The model under review builds one solid part; all positions refer to its coordinate system, in mm. Give positions to 0.01 mm unless a question says otherwise; leave off trailing zeros. Order: outer loops, then holes, each group sorted by start corner. A loop starts at its lowest first (then second) coordinate and runs counter-clockwise, first axis right, second up. Notation, with made-up numbers: (-34, 25.5) - (-8, 25.5) arc R37 cw to (-8, 62.5) - close; hole circle Ø11 at (67, 2.25). An arc over 180 degrees is marked (long way). Write item = value, one per line. Start each with the question number.
1. We need section B-B, the plane z = -0.6. State how many separate pieces and enclosed holes the cut face has, and give its area (3 significant figures).
2. For P1, Ø1.9, axis at x = -138.08, y = 6.57, coming from the -Z side; P2, Ø1.5, axis at x = 94.5, z = 0.5, coming from the -Y side; P3, Ø5, axis at x = 138.08, y = 6.57, coming from the -Z side; P4, Ø1.5, axis at x = 75, z = 0, coming from the +Y side, all flat-tipped, find the tip position at first contact; note any pin that passes through.
3. Wall thickness on probe 1 along Y at (x, z) = (49, 0.8); probe 2 along X at (y, z) = (-22.5, 0.15); probe 3 along Y at (x, z) = (-219, 1.2): over which ranges is each line inside the solid? List them lowest first.
4. We need section A-A, the plane y = -38.5. Give the boundary of the cut face in (x, z), and give its area (3 significant figures).
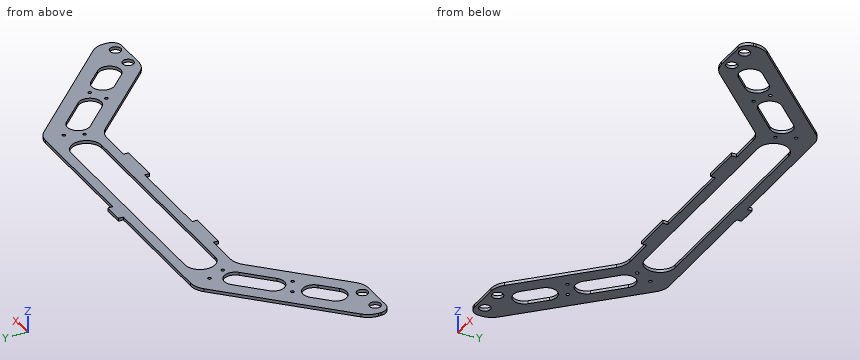
from build123d import *

# Parameters (mm, degrees)
SKETCH_1_R          = 5.5
EXTRUDE_1_DEPTH     = 1.5
CUT_EXTRUDE_6_DEPTH = 283.134941999
SKETCH_2_5_R        = 1.6
CUT_EXTRUDE_7_DEPTH = 283.134941999


with BuildPart() as part:
    # Sketch 1 → Extrude 1 (new, symmetric)
    with BuildSketch(Plane.XY):
        with BuildLine():
            Line((-125, 25), (-10, 25))
            Line((-10, 25), (-10, 30))
            Line((-10, 30), (10, 30))
            Line((10, 30), (10, 25))
            Line((10, 25), (125, 25))
            Line((125, 25), (137.426406871, 25))
            ThreePointArc((137.426406871, 25), (145.080075518, 23.47759065), (151.568542495, 19.142135624))
            Line((151.568542495, 19.142135624), (202.781745931, -32.071067812))
            Line((202.781745931, -32.071067812), (253.994949366, -83.284271247))
            ThreePointArc((253.994949366, -83.284271247), (258.330404393, -89.772738224), (259.852813742, -97.426406871))
            Line((259.852813742, -97.426406871), (259.852813742, -99.852813742))
            ThreePointArc((259.852813742, -99.852813742), (256.923881554, -106.923881554), (249.852813742, -109.852813742))
            Line((249.852813742, -109.852813742), (218.13708499, -109.852813742))
            ThreePointArc((218.13708499, -109.852813742), (210.483416343, -108.330404393), (203.994949366, -103.994949366))
            Line((203.994949366, -103.994949366), (130.857864376, -30.857864376))
            ThreePointArc((130.857864376, -30.857864376), (124.3693974, -26.52240935), (116.715728753, -25))
            Line((116.715728753, -25), (85, -25))
            Line((85, -25), (85, -30))
            Line((85, -30), (45, -30))
            Line((45, -30), (45, -25))
            Line((45, -25), (-45, -25))
            Line((-45, -25), (-45, -30))
            Line((-45, -30), (-85, -30))
            Line((-85, -30), (-85, -25))
            Line((-85, -25), (-116.715728753, -25))
            ThreePointArc((-116.715728753, -25), (-124.3693974, -26.52240935), (-130.857864376, -30.857864376))
            Line((-130.857864376, -30.857864376), (-203.994949366, -103.994949366))
            ThreePointArc((-203.994949366, -103.994949366), (-210.483416343, -108.330404393), (-218.13708499, -109.852813742))
            Line((-218.13708499, -109.852813742), (-249.852813742, -109.852813742))
            ThreePointArc((-249.852813742, -109.852813742), (-256.923881554, -106.923881554), (-259.852813742, -99.852813742))
            Line((-259.852813742, -99.852813742), (-259.852813742, -97.426406871))
            ThreePointArc((-259.852813742, -97.426406871), (-258.330404393, -89.772738224), (-253.994949366, -83.284271247))
            Line((-253.994949366, -83.284271247), (-202.781745931, -32.071067812))
            Line((-202.781745931, -32.071067812), (-151.568542495, 19.142135624))
            ThreePointArc((-151.568542495, 19.142135624), (-145.080075518, 23.47759065), (-137.426406871, 25))
            Line((-137.426406871, 25), (-125, 25))
        make_face()
        with Locations((-245.994949366, -101.352813742)):
            Circle(SKETCH_1_R, mode=Mode.SUBTRACT)
        with Locations((-221.994949366, -101.352813742)):
            Circle(SKETCH_1_R, mode=Mode.SUBTRACT)
        with Locations((221.994949366, -101.352813742)):
            Circle(SKETCH_1_R, mode=Mode.SUBTRACT)
        with Locations((245.994949366, -101.352813742)):
            Circle(SKETCH_1_R, mode=Mode.SUBTRACT)
    extrude(amount=EXTRUDE_1_DEPTH, both=True)

    # Sketch 2 → Cut-Extrude 6 (cut, through all)
    with BuildSketch(Plane.XY.offset(1.5)):
        with BuildLine():
            Line((-107.5, -15), (107.5, -15))
            ThreePointArc((107.5, -15), (122.5, 0), (107.5, 15))
            Line((107.5, 15), (-107.5, 15))
            ThreePointArc((-107.5, 15), (-122.5, 0), (-107.5, -15))
        make_face()
    extrude(amount=-CUT_EXTRUDE_6_DEPTH, mode=Mode.SUBTRACT)

    # Sketch 2_5 → Cut-Extrude 7 (cut, through all)
    with BuildSketch(Plane.XY.offset(1.5)):
        with Locations((-138.075378798, 6.566756826)):
            Circle(SKETCH_2_5_R)
        with Locations((-131.045941546, -10.403805922)):
            Circle(SKETCH_2_5_R)
        with Locations((-176.520445456, -55.878309832)):
            Circle(SKETCH_2_5_R)
        with Locations((-192.035164082, -47.393028458)):
            Circle(SKETCH_2_5_R)
        with Locations(Location((131.045941546, -10.403805922, 0), (0, 0, 180))):
            Circle(SKETCH_2_5_R)
        with Locations(Location((138.075378798, 6.566756826, 0), (0, 0, 180))):
            Circle(SKETCH_2_5_R)
        with Locations(Location((176.520445456, -55.878309832, 0), (0, 0, 180))):
            Circle(SKETCH_2_5_R)
        with Locations(Location((192.035164082, -47.393028458, 0), (0, 0, 180))):
            Circle(SKETCH_2_5_R)
        with BuildLine():
            Line((-141.060660172, -21.261670299), (-165.809397513, -46.01040764))
            ThreePointArc((-165.809397513, -46.01040764), (-181.365746699, -46.01040764), (-181.365746699, -30.454058454))
            Line((-181.365746699, -30.454058454), (-156.617009358, -5.705321112))
            ThreePointArc((-156.617009358, -5.705321112), (-141.060660172, -5.705321112), (-141.060660172, -21.261670299))
        make_face()
        with BuildLine():
            Line((-222.024386618, -71.112698372), (-207.882250994, -56.970562748))
            ThreePointArc((-207.882250994, -56.970562748), (-192.325901808, -56.970562748), (-192.325901808, -72.526911935))
            Line((-192.325901808, -72.526911935), (-206.468037432, -86.669047558))
            ThreePointArc((-206.468037432, -86.669047558), (-222.024386618, -86.669047558), (-222.024386618, -71.112698372))
        make_face()
        with BuildLine():
            Line((141.060660172, -21.261670299), (165.809397513, -46.01040764))
            ThreePointArc((165.809397513, -46.01040764), (181.365746699, -46.01040764), (181.365746699, -30.454058454))
            Line((181.365746699, -30.454058454), (156.617009358, -5.705321112))
            ThreePointArc((156.617009358, -5.705321112), (141.060660172, -5.705321112), (141.060660172, -21.261670299))
        make_face()
        with BuildLine():
            Line((222.024386618, -71.112698372), (207.882250994, -56.970562748))
            ThreePointArc((207.882250994, -56.970562748), (192.325901808, -56.970562748), (192.325901808, -72.526911935))
            Line((192.325901808, -72.526911935), (206.468037432, -86.669047558))
            ThreePointArc((206.468037432, -86.669047558), (222.024386618, -86.669047558), (222.024386618, -71.112698372))
        make_face()
    extrude(amount=-CUT_EXTRUDE_7_DEPTH, mode=Mode.SUBTRACT)


solid = part.part
Model answer:
q1.separate_pieces = 1
q1.enclosed_holes = 17
q1.area = 17,500 mm2
q2.P1 = through
q2.P2 = -25
q2.P3 = -1.5
q2.P4 = 25
q3.probe_1 = -30 to -15, 15 to 25
q3.probe_2 = -193.21 to -173.41, -142.3 to 142.3, 173.41 to 193.21
q3.probe_3 = -109.85 to -105.97, -96.74 to -88.81, -68.09 to -48.29
q4.outline = (-209.21, -1.5) - (-184.58, -1.5) - (-184.58, 1.5) - (-209.21, 1.5) - close; (-158.3, -1.5) - (-138.5, -1.5) - (-138.5, 1.5) - (-158.3, 1.5) - close; (138.5, -1.5) - (158.3, -1.5) - (158.3, 1.5) - (138.5, 1.5) - close; (184.58, -1.5) - (209.21, -1.5) - (209.21, 1.5) - (184.58, 1.5) - close
q4.area = 267 mm2
